```python
from build123d import *

# Parameters (mm, degrees)
SKETCH1_R           = 25.5
SKETCH1_R_2         = 23.5
BOSS_EXTRUDE1_DEPTH = 200


with BuildPart() as part:
    # Sketch1 → Boss-Extrude1 (new body)
    with BuildSketch(Plane(origin=(0, 0, 0), x_dir=(1, 0, 0), z_dir=(0, 1, 0))):
        Circle(SKETCH1_R)
        Circle(SKETCH1_R_2, mode=Mode.SUBTRACT)
    extrude(amount=BOSS_EXTRUDE1_DEPTH)

    # Sketch2 → Revolve1 (revolve)
    with BuildSketch(Plane.XY):
        with BuildLine():
            Line((-23.5, 0), (-5, 0))
            ThreePointArc((-5, 0), (-3.535533906, 3.535533906), (0, 5))
            Line((0, 5), (0, 7))
            ThreePointArc((0, 7), (-4.183300133, 5.61248608), (-6.708203932, 2))
            Line((-6.708203932, 2), (-23.5, 2))
            Line((-23.5, 2), (-23.5, 0))
        make_face()
    revolve(axis=Axis((0, 5, 0), (0, 1, 0)))


solid = part.part
```
Check sheet for the modelled part. Datum: model origin and axes. Units: mm. A direction names the side the tool comes from. Round coordinates to 2 decimals unless told otherwise and drop trailing zeros. Order: outer loops, then holes, each group sorted by start corner. A loop starts at its lowest first (then second) coordinate and runs counter-clockwise, first axis right, second up.
1) Mould release check, pull along Z, two halves, no side actions. Record for faces 1 (the flat face through (11, 200, 21)), 2 (the cylindrical face through (22.4, 99.6, -7.1)), 3 (the cylindrical face through (-5.5, 98.6, 24.9)): +Z half, -Z half, draft (parallel to the pull), parting line (faces both ways), or undercut.
2) Section check D-D (x = -10.5). Record the boundary of the cut face in (y, z).
3) Section check B-B (x = 2.5). Record the boundary of the cut face in (y, z), and give its area (3 significant figures).
4) Go/stop test with flat-tipped pins: pin 1 Ø12 at (x, y) = (9, 161.5) entering from +Z; pin 2 Ø8 at (x, y) = (-12, 46) entering from -Z; pin 3 Ø3 at (y, z) = (124.5, 13.5) entering from +X. Record where each tip stops, or that it passes through.
5) Scan lines: line 1 (Z direction, x = 0, y = 85); line 2 (X direction, y = 12.5, z = -9.5). Record each from-to range of solid material in increasing order.
6) Tool access check on faces 4 (the flat face through (-5.3, 0, 0.4)), 5 (the flat face through (5, 2, -5)). Record the directions out of +Z, -Z, +X, -X, +Y, -Y that give a thin tool (end or side, any length) a straight path to the whole face; none if there is none.
7) Section check A-A (z = 0). Record the boundary of the cut face in (x, y), and give its area (3 significant figures).
8) Section check C-C (y = 98). Record the boundary of the cut face in (x, z).
Result:
1. face 1: draft
1. face 2: undercut
1. face 3: parting line
2. outline: (0, -23.24) - (200, -23.24) - (200, -21.02) - (2, -21.02) - (2, 21.02) - (200, 21.02) - (200, 23.24) - (0, 23.24) - close
3. outline: (0, -25.38) - (200, -25.38) - (200, -23.37) - (2, -23.37) - (2, -6.22) arc R6.54 ccw to (2, 6.22) - (2, 23.37) - (200, 23.37) - (200, 25.38) - (0, 25.38) - (0, 4.33) arc R4.33 cw to (0, -4.33) - close
3. area: 910 mm2
4. pin 1: stops at z = 25.32
4. pin 2: stops at z = -24.21
4. pin 3: stops at x = 22.5
5. line 1: z = -25.5 to -23.5, 23.5 to 25.5
5. line 2: x = -23.66 to -21.49, 21.49 to 23.66
6. face 4: +Z, -Z, +X, -X, -Y
6. face 5: +Y
7. outline: (-25.5, 0) - (-5, 0) arc R5 cw to (5, 0) - (25.5, 0) - (25.5, 200) - (23.5, 200) - (23.5, 2) - (6.71, 2) arc R7 ccw to (-6.71, 2) - (-23.5, 2) - (-23.5, 200) - (-25.5, 200) - close
7. area: 904 mm2
8. outline: circle Ø51 at (0, 0); hole circle Ø47 at (0, 0)
